Design review of the part built by this model. Coordinates are the model's own, in mm. Face numbers are marked on the shaded views. Coordinates: 2 decimals unless noted, no trailing zeros. Order: outer loops, then holes, each group sorted by start corner. A loop starts at its lowest first (then second) coordinate and runs counter-clockwise, first axis right, second up. Notation, with made-up numbers: (15.5, -15) -> (21.5, -15) arc R15 cw to (21.5, -4) -> close; hole circle Ø3 at (80, -21). An arc over 180 degrees is marked (long way). Use a Markdown table: item, result. Add a question column.
Q1. The part is to be moulded in two halves that separate along Z. For the marked faces 1, 2 and 3, say which applies: pulls with the +Z half, pulls with the -Z half, needs draft (parallel to the pull), parting line crosses it, or undercut.
Q2. Add section A-A (y = 49.5). State the section outline as (x, z) points.
Q3. Wall thickness on probe 1 along Z at (x, y) = (-21, 85); probe 2 along Z at (x, y) = (15.5, 50.5); probe 3 along Y at (x, z) = (4.5, 38): over which ranges is each line inside the solid? List them lowest first.
Q4. Add section D-D (x = 2.5). Count the separate pieces of the cut face and the enclosed holes in it, then the cut area to 3 significant figures.
Q5. Add section C-C (y = 1). State the section outline as (x, z) points, then the cut area to 3 significant figures.
Q6. Insertion check: pin 1 (11 mm diameter, centred on y = 4, z = 189.5, fed in from +X); pin 2 (8 mm diameter, centred on x = -21.5, y = 54.5, fed in from -Z); pin 3 (11 mm diameter, centred on y = 13.5, z = 5, fed in from -X); pin 4 (10 mm diameter, centred on x = -17, z = 58, fed in from -Y). Each pin has a flat end and moves straight along its axis. Give the tip position at first contact, or say it passes through.
Q7. Add section B-B (x = -22.5). State the section outline as (y, z) points.
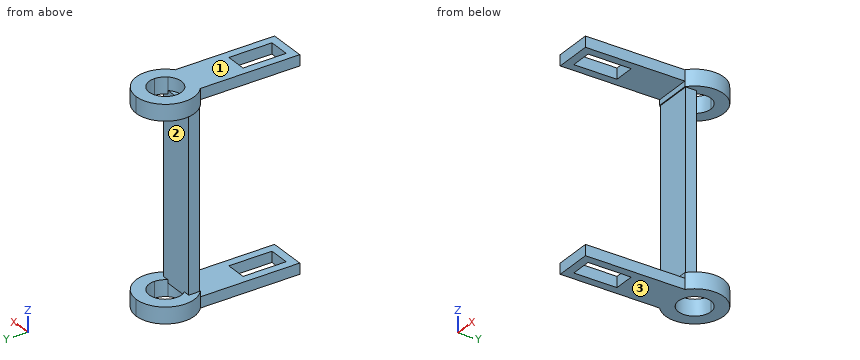
from build123d import *
from build123d.topology import SkipClean

# Parameters (mm, degrees)
ESQUISSE1_W             = 34.5
ESQUISSE1_H             = 55
ESQUISSE1_W_2           = 19.5
ESQUISSE1_H_2           = 40
BOSS_EXTRU_1_DEPTH      = 10
ESQUISSE6_W             = 34.5
ESQUISSE6_H             = 10
BOSS_EXTRU_2_DEPTH      = 48
ESQUISSE7_W             = 34.5
ESQUISSE7_H             = 10
BOSS_EXTRU_3_DEPTH      = 87.5
BOSS_EXTRU_4_DEPTH      = 15
ESQUISSE9_R             = 15
ENL_V_MAT_EXTRU_1_DEPTH = 12
BOSS_EXTRU_5_REACH      = 231.433
BOSS_EXTRU_5_END_RADIUS = 27
ESQUISSE10_W            = 5
ESQUISSE10_H            = 0.771073636


with BuildPart() as part:
    # Esquisse1 → Boss.-Extru.1 (new body)
    with BuildSketch(Plane.XY):
        Rectangle(ESQUISSE1_W, ESQUISSE1_H)
        Rectangle(ESQUISSE1_W_2, ESQUISSE1_H_2, mode=Mode.SUBTRACT)
    boss_extru_1 = extrude(amount=BOSS_EXTRU_1_DEPTH)

    # Esquisse6 → Boss.-Extru.2 (add)
    with BuildSketch(Plane(origin=(0, 27.5, 0), x_dir=(1, 0, 0), z_dir=(0, 1, 0))):
        with Locations((0, -5)):
            Rectangle(ESQUISSE6_W, ESQUISSE6_H)
    boss_extru_2 = extrude(amount=BOSS_EXTRU_2_DEPTH)

    # Esquisse7 → Boss.-Extru.3 (add)
    with BuildSketch(Plane.XY.offset(10)):
        with Locations((0, 70.5)):
            Rectangle(ESQUISSE7_W, ESQUISSE7_H)
    boss_extru_3 = extrude(amount=BOSS_EXTRU_3_DEPTH)

    # Symétrie1: Boss.-Extru.1, Boss.-Extru.2, Boss.-Extru.3 across plane
    add(boss_extru_1.mirror(Plane(origin=(0, 0, 97.5), x_dir=(1, 0, 0), z_dir=(0, 0, -1))))
    add(boss_extru_2.mirror(Plane(origin=(0, 0, 97.5), x_dir=(1, 0, 0), z_dir=(0, 0, -1))))
    add(boss_extru_3.mirror(Plane(origin=(0, 0, 97.5), x_dir=(1, 0, 0), z_dir=(0, 0, -1))))

    # Esquisse8 → Boss.-Extru.4 (add)
    with BuildSketch(Plane.XY.offset(195)):
        with BuildLine():
            Line((11.180339887, 75.5), (17.25, 75.5))
            Line((17.25, 75.5), (17.25, 64.728926364))
            ThreePointArc((17.25, 64.728926364), (25.395068302, 94.670087563), (0, 112.5))
            Line((0, 112.5), (0, 100.5))
            ThreePointArc((0, 100.5), (10.606601718, 96.106601718), (15, 85.5))
            ThreePointArc((15, 85.5), (14.012585384, 80.147668653), (11.180339887, 75.5))
        make_face()
        with BuildLine():
            Line((0, 100.5), (0, 112.5))
            ThreePointArc((0, 112.5), (-25.395068302, 94.670087563), (-17.25, 64.728926364))
            Line((-17.25, 64.728926364), (-17.25, 75.5))
            Line((-17.25, 75.5), (-11.180339887, 75.5))
            ThreePointArc((-11.180339887, 75.5), (-13.693063938, 91.623724357), (0, 100.5))
        make_face()
    boss_extru_4 = extrude(amount=-BOSS_EXTRU_4_DEPTH)

    # Esquisse9 → Enlèv. mat.-Extru.1 (cut)
    with SkipClean():  # the faces are left unmerged after this step: merging them gives an invalid solid
        with BuildSketch(Plane.XY.offset(195)):
            with Locations((0, 85.5)):
                Circle(ESQUISSE9_R)
        enl_v_mat_extru_1 = extrude(amount=-ENL_V_MAT_EXTRU_1_DEPTH, mode=Mode.SUBTRACT)

    # Boss.-Extru.5: up to this cylinder (the profile starts inside it)
    with SkipClean():  # the faces are left unmerged after this step: merging them gives an invalid solid
        boss_extru_5_end = Plane(origin=(0, 85.5, 182.5), z_dir=(0, 0, 1)) * Cylinder(BOSS_EXTRU_5_END_RADIUS, 517.866, mode=Mode.PRIVATE)
        # Esquisse10 → Boss.-Extru.5 (add, up to the surface)
        with BuildSketch(Plane.ZY.offset(-17.25), mode=Mode.PRIVATE) as boss_extru_5_sk1:
            with Locations((182.5, 65.114463182)):
                Rectangle(ESQUISSE10_W, ESQUISSE10_H)
        boss_extru_5_tool1 = extrude(boss_extru_5_sk1.sketch, amount=BOSS_EXTRU_5_REACH, mode=Mode.PRIVATE) & boss_extru_5_end
        boss_extru_5 = boss_extru_5_tool1.solids().sort_by_distance((17.25, 65.114463, 182.5))[0]
        add(boss_extru_5)

    # Symétrie2: Boss.-Extru.4, Enlèv. mat.-Extru.1, Boss.-Extru.5 across plane
    with SkipClean():  # the faces are left unmerged after this step: merging them gives an invalid solid
        add(boss_extru_4.mirror(Plane(origin=(0, 0, 97.5), x_dir=(1, 0, 0), z_dir=(0, 0, -1))))
        add(enl_v_mat_extru_1.mirror(Plane(origin=(0, 0, 97.5), x_dir=(1, 0, 0), z_dir=(0, 0, -1))), mode=Mode.SUBTRACT)
        add(boss_extru_5.mirror(Plane(origin=(0, 0, 97.5), x_dir=(1, 0, 0), z_dir=(0, 0, -1))))


solid = part.part
Established:
| question | item | result |
|---|---|---|
| 1 | face 1 | pulls with the +Z half |
| 1 | face 2 | undercut |
| 1 | face 3 | pulls with the -Z half |
| 2 | outline | (-17.25, 0) -> (17.25, 0) -> (17.25, 10) -> (-17.25, 10) -> close; (-17.25, 185) -> (17.25, 185) -> (17.25, 195) -> (-17.25, 195) -> close |
| 3 | probe 1 | 0 to 15, 180 to 195 |
| 3 | probe 2 | 0 to 10, 185 to 195 |
| 3 | probe 3 | 65.5 to 75.5 |
| 4 | separate pieces | 5 |
| 4 | enclosed holes | 0 |
| 4 | area | 3,270 mm^2 |
| 5 | outline | (-17.25, 0) -> (-9.75, 0) -> (-9.75, 10) -> (-17.25, 10) -> close; (-17.25, 185) -> (-9.75, 185) -> (-9.75, 195) -> (-17.25, 195) -> close; (9.75, 0) -> (17.25, 0) -> (17.25, 10) -> (9.75, 10) -> close; (9.75, 185) -> (17.25, 185) -> (17.25, 195) -> (9.75, 195) -> close |
| 5 | area | 300 mm^2 |
| 6 | pin 1 | x = 17.25 |
| 6 | pin 2 | through |
| 6 | pin 3 | x = -17.25 |
| 6 | pin 4 | y = 65.5 |
| 7 | outline | (70.58, 0) -> (100.42, 0) -> (100.42, 15) -> (70.58, 15) -> close; (70.58, 180) -> (100.42, 180) -> (100.42, 195) -> (70.58, 195) -> close |
